Check sheet for the modelled part. Datum: model origin and axes. Units: mm. A direction names the side the tool comes from. Round coordinates to 2 decimals unless told otherwise and drop trailing zeros. Write each loop counter-clockwise with the first axis right and the second up, starting at its lowest first coordinate (ties: lowest second). Pieces come first, ordered by that corner, then holes. Notation, with made-up numbers: (58.25, 53.25) -> (64.25, 53.25) arc R15 cw to (64.25, 73.25) -> close; hole circle Ø2 at (-26.5, -0.5). An arc over 180 degrees is marked (long way). Put each result on its own line as item: value. Start each with the question number.
from build123d import *

# Parameters (mm, degrees)
SKETCH1_W                         = 19.05
SKETCH1_H                         = 19.05
BOSS_EXTRUDE1_DEPTH               = 38.1
F_1_4_20_TAPPED_HOLE1_D           = 5.1054
F_1_4_20_TAPPED_HOLE1_DEPTH       = 25.4
F_1_4_20_TAPPED_HOLE1_CSINK_D     = 7.62
F_1_4_20_TAPPED_HOLE1_CSINK_ANGLE = 100
F_1_4_20_TAPPED_HOLE1_TIP         = 1.533816902
FILLET1_R                         = 5.08


with BuildPart() as part:
    # Sketch1 → Boss-Extrude1 (new body)
    with BuildSketch(Plane(origin=(0, 0, 0), x_dir=(1, 0, 0), z_dir=(0, 1, 0))):
        Rectangle(SKETCH1_W, SKETCH1_H)
    extrude(amount=BOSS_EXTRUDE1_DEPTH)

    # 1/4-20 Tapped Hole1
    with Locations(Plane(origin=(0, 38.1, 0), x_dir=(1, 0, 0), z_dir=(0, 1, 0))):
        with Locations((0, 0)):
            CounterSinkHole(F_1_4_20_TAPPED_HOLE1_D / 2, F_1_4_20_TAPPED_HOLE1_CSINK_D / 2, depth=F_1_4_20_TAPPED_HOLE1_DEPTH, counter_sink_angle=F_1_4_20_TAPPED_HOLE1_CSINK_ANGLE)
            with Locations((0, 0, -(F_1_4_20_TAPPED_HOLE1_DEPTH + F_1_4_20_TAPPED_HOLE1_TIP / 2))):  # 118° drill point
                Cone(0, F_1_4_20_TAPPED_HOLE1_D / 2, F_1_4_20_TAPPED_HOLE1_TIP, mode=Mode.SUBTRACT)

    # Fillet1
    fillet1_edges = [part.edges().sort_by_distance(p)[0] for p in [
        (9.525, 19.05, 9.525),
        (-9.525, 19.05, 9.525),
        (-9.525, 19.05, -9.525),
        (9.525, 19.05, -9.525),
    ]]
    fillet(fillet1_edges, radius=FILLET1_R)


solid = part.part
1. Material ranges on L1, parallel to Z at x = 0, y = 27 (3 decimals); L2, parallel to X at y = 26.5, z = -4.75; L3, parallel to Z at x = 0.5, y = 33 (3 decimals), recorded low to high. Write a range as [from, to].
2. Access from +Z, -Z, +X, -X, +Y, -Y to the whole of each face (thin tool, end or side, straight path). Record for faces 1 (the cylindrical face through (-2.435, 24.702, -0.767)), 2 (the flat face through (0, 19, 9.525)).
3. Section check C-C, the plane z = 7.25. Enter the section's corners in (x, y), then the cut area to 3 significant figures.
4. Draft check along X on faces 3 (the conical face through (0.41, 11.433, 0.17)), 4 (the flat face through (4, 38.1, 0)), 5 (the flat face through (-9.525, 19, 0)). Enter one of: released by +X, released by -X, zero draft, split by the parting line, or undercut.
5. Section check B-B, the plane y = 5.5. Enter the section's corners in (x, z) (3 decimals), then the cut area to 3 significant figures.
6. Section check D-D, the plane x = -6.75. Enter the section's corners in (y, z), then the cut area to 3 significant figures.
7. Gauge pin test, flat end, axial feed: P1, Ø5, axis at x = 7, y = 14, coming from the +Z side. Record the tip position at first contact, or that the pin passes through.
8. Section check A-A, the plane y = 21.5. Enter the section's corners in (x, z) (3 decimals).
Reply:
1. L1: z = [-9.525, -2.553], [2.553, 9.525]
1. L2: x = [-9.52, 9.52]
1. L3: z = [-9.525, -2.503], [2.503, 9.525]
2. face 1: +Y
2. face 2: +Z, +X, -X, +Y, -Y
3. outline: (-8.68, 0) -> (8.68, 0) -> (8.68, 38.1) -> (-8.68, 38.1) -> close
3. area: 661 mm2
4. face 3: undercut
4. face 4: zero draft
4. face 5: released by -X
5. outline: (-9.525, -4.445) arc R5.08 ccw to (-4.445, -9.525) -> (4.445, -9.525) arc R5.08 ccw to (9.525, -4.445) -> (9.525, 4.445) arc R5.08 ccw to (4.445, 9.525) -> (-4.445, 9.525) arc R5.08 ccw to (-9.525, 4.445) -> close
5. area: 341 mm2
6. outline: (0, -8.97) -> (38.1, -8.97) -> (38.1, 8.97) -> (0, 8.97) -> close
6. area: 684 mm2
7. P1: stops at z = 9.52
8. outline: (-9.525, -4.445) arc R5.08 ccw to (-4.445, -9.525) -> (4.445, -9.525) arc R5.08 ccw to (9.525, -4.445) -> (9.525, 4.445) arc R5.08 ccw to (4.445, 9.525) -> (-4.445, 9.525) arc R5.08 ccw to (-9.525, 4.445) -> close; hole circle Ø5.105 at (0, 0)
